Input: part model. Units: mm. Frame: model coordinates. Face numbers are marked on the shaded views. Give positions to 0.01 mm unless a question says otherwise; leave off trailing zeros. Order: outer loops, then holes, each group sorted by start corner. A loop starts at its lowest first (then second) coordinate and runs counter-clockwise, first axis right, second up. Notation, with made-up numbers: M 64.5,-34.75 L 105.5,-34.75 A18 ccw 105.5,0.25 Z; hole C 34.5,45 d6. An arc over 180 degrees is marked long. Use a Markdown table: item, result.
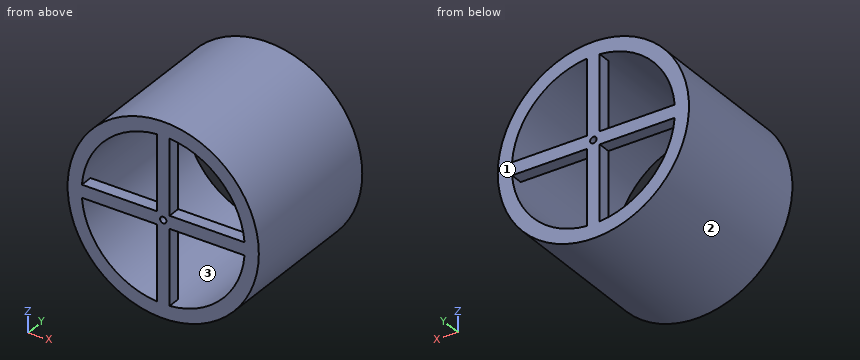
from build123d import *

# Parameters (mm, degrees)
F0_R     = 190.75
F0_R_2   = 162.7125
F1_DEPTH = 304.8
F3_DEPTH = 25.4
F5_DEPTH = 25.4
F6_R     = 6.35
F7_DEPTH = 382


with BuildPart() as f1:
    # F0 (on Front) → F1 (new body)
    with BuildSketch(Plane.XZ):
        Circle(F0_R)
        Circle(F0_R_2, mode=Mode.SUBTRACT)
    extrude(amount=F1_DEPTH)

    # F2 (on face) → F3 (join)
    with BuildSketch(Plane.XZ.offset(304.8)):
        with BuildLine():
            ThreePointArc((12.7, 162.216114), (0, 162.7125), (-12.7, 162.216114))
            Line((-12.7, 162.216114), (-12.7, 12.7))
            Line((-12.7, 12.7), (-12.7, -12.7))
            Line((-12.7, -12.7), (-12.7, -162.216114))
            ThreePointArc((-12.7, -162.216114), (0, -162.7125), (12.7, -162.216114))
            Line((12.7, -162.216114), (12.7, -12.7))
            Line((12.7, -12.7), (12.7, 12.7))
            Line((12.7, 12.7), (12.7, 162.216114))
        make_face()
        with BuildLine():
            Line((-12.7, -12.7), (-12.7, 12.7))
            Line((-12.7, 12.7), (-162.216114, 12.7))
            ThreePointArc((-162.216114, 12.7), (-162.7125, 0), (-162.216114, -12.7))
            Line((-162.216114, -12.7), (-12.7, -12.7))
        make_face()
        with BuildLine():
            Line((162.216114, 12.7), (12.7, 12.7))
            Line((12.7, 12.7), (12.7, -12.7))
            Line((12.7, -12.7), (162.216114, -12.7))
            ThreePointArc((162.216114, -12.7), (162.7125, 0), (162.216114, 12.7))
        make_face()
        with BuildLine():
            Line((162.216114, 12.7), (12.7, 12.7))
            Line((12.7, 12.7), (12.7, -12.7))
            Line((12.7, -12.7), (162.216114, -12.7))
            ThreePointArc((162.216114, -12.7), (162.588356, -6.354849), (162.7125, 0))
            ThreePointArc((162.7125, 0), (162.588356, 6.354849), (162.216114, 12.7))
        make_face()
    extrude(amount=-F3_DEPTH)

    # F4 (on face) → F5 (join)
    with BuildSketch(Plane(origin=(0, 0, 0), x_dir=(-1, 0, 0), z_dir=(0, 1, 0))):
        with BuildLine():
            Line((-12.7, 162.216114), (-12.7, 12.7))
            Line((-12.7, 12.7), (-162.216114, 12.7))
            ThreePointArc((-162.216114, 12.7), (-162.7125, 0), (-162.216114, -12.7))
            Line((-162.216114, -12.7), (-12.7, -12.7))
            Line((-12.7, -12.7), (-12.7, -162.216114))
            ThreePointArc((-12.7, -162.216114), (0, -162.7125), (12.7, -162.216114))
            Line((12.7, -162.216114), (12.7, -12.7))
            Line((12.7, -12.7), (162.216114, -12.7))
            ThreePointArc((162.216114, -12.7), (162.588356, -6.354849), (162.7125, 0))
            ThreePointArc((162.7125, 0), (162.588356, 6.354849), (162.216114, 12.7))
            Line((162.216114, 12.7), (12.7, 12.7))
            Line((12.7, 12.7), (12.7, 162.216114))
            ThreePointArc((12.7, 162.216114), (0, 162.7125), (-12.7, 162.216114))
        make_face()
    extrude(amount=-F5_DEPTH)

    # F6 (on face) → F7 (cut)
    with BuildSketch(Plane(origin=(0, 0, 0), x_dir=(-1, 0, 0), z_dir=(0, 1, 0))):
        Circle(F6_R)
    extrude(amount=-F7_DEPTH, mode=Mode.SUBTRACT)


solid = f1.part
1) Cut plane D-D on x = 46. Return loops of the section in (y, z), and give its area (3 significant figures).
Response values:
| item | result |
|---|---|
| outline | M -304.8,-185.12 L 0,-185.12 L 0,-156.07 L -304.8,-156.07 Z; M -304.8,-12.7 L -279.4,-12.7 L -279.4,12.7 L -304.8,12.7 Z; M -304.8,156.07 L 0,156.07 L 0,185.12 L -304.8,185.12 Z; M -25.4,-12.7 L 0,-12.7 L 0,12.7 L -25.4,12.7 Z |
| area | 19,000 mm² |
2) Material intervals for line 1 (Z direction, x = 0, y = -221.5); line 2 (Z direction, x = 0, y = -296); line 3 (X direction, y = -19, z = -60), sorted ascending. Write a range as from..to.
Response values:
| item | result |
|---|---|
| line 1 | z = -190.75..-162.71, 162.71..190.75 |
| line 2 | z = -190.75..-6.35, 6.35..190.75 |
| line 3 | x = -181.07..-151.25, -12.7..12.7, 151.25..181.07 |
3) Cut plane A-A on z = 0. Return loops of the section in (x, y).
Response values:
| item | result |
|---|---|
| outline | M -190.75,-304.8 L -6.35,-304.8 L -6.35,-279.4 L -162.71,-279.4 L -162.71,-25.4 L -6.35,-25.4 L -6.35,0 L -190.75,0 Z; M 6.35,-304.8 L 190.75,-304.8 L 190.75,0 L 6.35,0 L 6.35,-25.4 L 162.71,-25.4 L 162.71,-279.4 L 6.35,-279.4 Z |
4) Cut plane C-C on z = 65. Return loops of the section in (x, y), and give its area (3 significant figures).
Response values:
| item | result |
|---|---|
| outline | M -179.33,-304.8 L -149.17,-304.8 L -149.17,0 L -179.33,0 Z; M -12.7,-304.8 L 12.7,-304.8 L 12.7,-279.4 L -12.7,-279.4 Z; M -12.7,-25.4 L 12.7,-25.4 L 12.7,0 L -12.7,0 Z; M 149.17,-304.8 L 179.33,-304.8 L 179.33,0 L 149.17,0 Z |
| area | 19,700 mm² |
5) Mould query, pull axis X, two halves, no side actions, for the marked faces 1, 2 and 3. Classes: released by +X, released by -X, zero draft, split by the parting line, or undercut.
Response values:
| item | result |
|---|---|
| face 1 | zero draft |
| face 2 | split by the parting line |
| face 3 | undercut |
6) First-contact query: pin 1 Ø8 at (x, y) = (133.5, -105) entering from +Z; pin 2 Ø12 at (y, z) = (-113.5, -80) entering from -X; pin 3 Ø12.5 at (x, y) = (71, -11.5) entering from +Z. Flat tips, straight axial feed; report the tip coordinate or a pass-through.
Response values:
| item | result |
|---|---|
| pin 1 | stops at z = 140.05 |
| pin 2 | stops at x = -175.81 |
| pin 3 | stops at z = 179.42 |
7) Cut plane B-B on x = 0. Return loops of the section in (y, z), and give its area (3 significant figures).
Response values:
| item | result |
|---|---|
| outline | M -304.8,-190.75 L 0,-190.75 L 0,-6.35 L -25.4,-6.35 L -25.4,-162.71 L -279.4,-162.71 L -279.4,-6.35 L -304.8,-6.35 Z; M -304.8,6.35 L -279.4,6.35 L -279.4,162.71 L -25.4,162.71 L -25.4,6.35 L 0,6.35 L 0,190.75 L -304.8,190.75 Z |
| area | 33,000 mm² |
